Job drawing, mm, ordinate dimensions from the low corner. One solid piece. A direction names the side the tool comes from. Give positions to 0.01 mm unless a question says otherwise; leave off trailing zeros. Loops run counter-clockwise (first coordinate to the right, second up) from the corner with the lowest first, then second, coordinate; pieces in that order, holes last. Notation, with made-up numbers: M 17,-34 L 56,-34 A21 cw 56,-22 Z; hole C -12.75,73.5 d3. An arc over 180 degrees is marked long. Put each result on its own line as item: value.
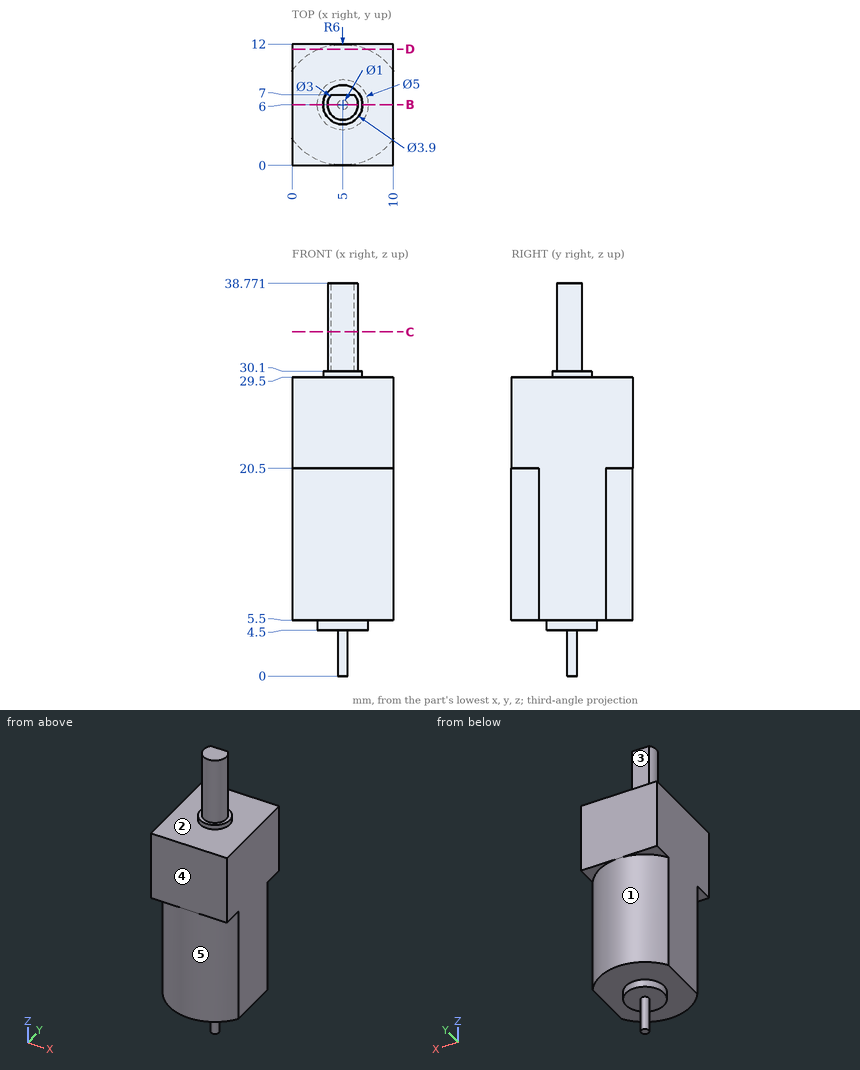
Q1. Drop flat-ended pins along their axis: pin 1 Ø3 at (x, y) = (7, 7.5) entering from -Z; pin 2 Ø1.1 at (x, z) = (4.5, 34) entering from +Y; pin 3 Ø4 at (y, z) = (10.5, 34.5) entering from -X; pin 4 Ø1.3 at (x, y) = (7, 10) entering from -Z. Give the stop position or say it passes through.
Here are the results:
pin 1: z = 4.5
pin 2: y = 7
pin 3: through
pin 4: z = 5.5
Q2. Probe line 1 (Z direction, x = 1.25, y = 2.75); line 2 (Z direction, x = 3.5, y = 5.5); line 3 (X direction, y = 6.75, z = 34.5). List the from-to ranges inside material, lowest first. Write a range as from..to.
Here are the results:
line 1: 5.5..29.5
line 2: 4.5..30.1
line 3: 3.7..6.3
Q3. Tool access for the marked faces 1, 2, 3, 4 and 5: list every direction of +Z, -Z, +X, -X, +Y, -Y with a clear straight run to the whole face (end or side of a thin tool).
Here are the results:
face 1: -Z, +Y
face 2: +Z
face 3: +Z, +X, -X, +Y
face 4: +Z, -Z, +X, -X, -Y
face 5: -Z, -Y
Q4. Slice it at D-D (y = 11.5). List the corners of the cut face in (x, z).
Here are the results:
outline: M 0,20.5 L 2.6,20.5 L 2.6,5.5 L 7.4,5.5 L 7.4,20.5 L 10,20.5 L 10,29.5 L 0,29.5 Z
Q5. Slice it at C-C (z = 34). List the corners of the cut face in (x, y).
Here are the results:
outline: M 3.88,7 A1.5 ccw long 6.12,7 Z
Q6. Slice it at B-B (y = 6). List the corners of the cut face in (x, z), and give its area (3 significant figures).
Here are the results:
outline: M 0,5.5 L 2.5,5.5 L 2.5,4.5 L 4.5,4.5 L 4.5,0 L 5.5,0 L 5.5,4.5 L 7.5,4.5 L 7.5,5.5 L 10,5.5 L 10,29.5 L 6.95,29.5 L 6.95,30.1 L 6.5,30.1 L 6.5,38.77 L 3.5,38.77 L 3.5,30.1 L 3.05,30.1 L 3.05,29.5 L 0,29.5 Z
area: 278 mm²
